CAD build for the part. Positions are in the model's coordinates, mm. A direction names the side the tool comes from. Round coordinates to 2 decimals unless told otherwise and drop trailing zeros. Loops run counter-clockwise (first coordinate to the right, second up) from the corner with the lowest first, then second, coordinate; pieces in that order, holes last. Notation, with made-up numbers: M 78.25,83 L 85.25,83 A21 cw 85.25,103 Z; hole C 42,82 d5. An arc over 180 degrees is marked long. Use one line per item in the form item = value.
from build123d import *

# Parameters (mm, degrees)
F0_W      = 4876.8
F0_H      = 1066.8
F1_DEPTH  = 101.6
F3_DEPTH  = 1016
F7_W      = 3860.8
F7_H      = 1066.8
F8_DEPTH  = 458.42061
F9_W      = 1016
F9_H      = 939.8
F10_DEPTH = 457.2


# Not quite as in the source:
# - a feature of the source that left no trace in its solid (it failed there, or was rolled back) is left out


with BuildPart() as f1:
    # F0 (on Top) → F1 (new body)
    with BuildSketch(Plane.XY):
        Rectangle(F0_W, F0_H)
    extrude(amount=-F1_DEPTH)

    # F2 (on face) → F3 (join)
    with BuildSketch(Plane(origin=(-2438.4, 0, 0), x_dir=(0, -1, 0), z_dir=(-1, 0, 0))):
        Polygon((533.4, -187.96), (533.4, 0), (304.8, 0), (-533.4, 0), (-533.4, -939.8), (304.8, -939.8), (1447.8, -939.8), (1447.8, -751.84), (1219.2, -751.84), (1219.2, -563.88), (990.6, -563.88), (990.6, -375.92), (762, -375.92), (762, -187.96), align=None)
    extrude(amount=-F3_DEPTH)

    # F7 (on face) → F8 (cut)
    with BuildSketch(Plane.XY):
        with Locations((508, 0)):
            Rectangle(F7_W, F7_H)
    extrude(amount=-F8_DEPTH, mode=Mode.SUBTRACT)

    # F9 (on face) → F10 (join)
    with BuildSketch(Plane(origin=(0, 533.4, 0), x_dir=(-1, 0, 0), z_dir=(0, 1, 0))):
        with Locations((1930.4, -469.9)):
            Rectangle(F9_W, F9_H)
    extrude(amount=F10_DEPTH)


solid = f1.part
1. Cut at B-B on z = -643. Write the cut outline in (x, y).
Completed:
outline = M -2438.4,-1219.2 L -1422.4,-1219.2 L -1422.4,990.6 L -2438.4,990.6 Z
2. Probe line 1 along Y through (x, z) = (-1863, -166); line 2 along Y through (x, z) = (-2237, -383); line 3 along Z through (x, y) = (-1644, -598). List the from-to ranges inside material, lowest first. Write a range as from..to.
Completed:
line_1 = -533.4..990.6
line_2 = -990.6..990.6
line_3 = -939.8..-187.96
3. Cut at C-C on y = -591. Write the cut outline in (x, z), and give its area (3 significant figures).
Completed:
outline = M -2438.4,-939.8 L -1422.4,-939.8 L -1422.4,-187.96 L -2438.4,-187.96 Z
area = 764,000 mm2
4. Tool access for faces 1 (the face through (-1923, 218, 0)), 2 (the face through (-1938, -878, -375.92)): list every direction of +Z, -Z, +X, -X, +Y, -Y with a clear straight run to the whole face (end or side of a thin tool).
Completed:
face_1 = +Z, +X, -X, +Y, -Y
face_2 = +Z, +X, -X, -Y
5. Cut at A-A on x = -2175. Write the cut outline in (y, z), and give its area (3 significant figures).
Completed:
outline = M -1447.8,-939.8 L 990.6,-939.8 L 990.6,0 L -533.4,0 L -533.4,-187.96 L -762,-187.96 L -762,-375.92 L -990.6,-375.92 L -990.6,-563.88 L -1219.2,-563.88 L -1219.2,-751.84 L -1447.8,-751.84 Z
area = 1,860,000 mm2
6. Drop a flat-ended pin along its axis: P1, Ø10, axis at x = -2151.5, z = -402, coming from the -Y side. Give the stop position or say it passes through.
Completed:
P1 = -990.6
